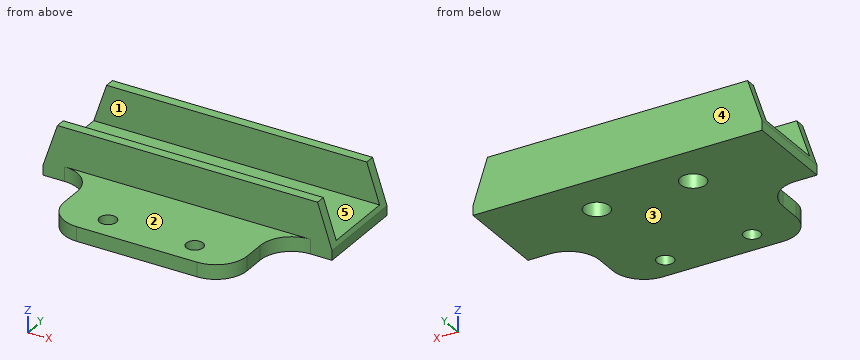
Autodesk Fusion 360 part; units mm, degrees
sketch "Esquisse1" plane through (0, 0, 0) normal (0, 0, 1) x (1, 0, 0)
  line L0 (0, 0) -> (60, 0)
  line L1 (60, 0) -> (60, 36.5)
  line L2 (60, 36.5) -> (0, 36.5)
  line L3 (0, 36.5) -> (0, 0)
  line L4 (0, 5) -> (60, 5) construction
  line L5 (0, 33.5) -> (60, 33.5) construction
  circle A0 centre (21, 5) radius 1.75
  circle A1 centre (39, 5) radius 1.75
  dimension "d1" = 28.5
  dimension "d2" = 60
  dimension "d3" = 18
  dimension "d4" = 21
  dimension "d5" = 3.5
  dimension "d6" = 5
  dimension "d7" = 3
extrude "Extrusion1" add sketch "Esquisse1" along normal blind 3
sketch "Esquisse2" plane through (0, 0, 3) normal (0, 0, 1) x (1, 0, 0)
  circle A0 centre (39, 5) radius 1.75
  circle A1 centre (21, 5) radius 1.75
  line L0 (0, 36.5) -> (0, 0)
  line L1 (0, 0) -> (60, 0)
  line L2 (60, 0) -> (60, 36.5)
  line L3 (60, 36.5) -> (0, 36.5)
  line L4 (0, 36.5) -> (60, 36.5)
  line L5 (60, 36.5) -> (60, 34.5)
  line L6 (60, 34.5) -> (0, 34.5)
  line L7 (0, 34.5) -> (0, 36.5)
  line L8 (0, 17.5) -> (60, 17.5)
  line L9 (60, 17.5) -> (60, 19.5)
  line L10 (60, 19.5) -> (0, 19.5)
  line L11 (0, 19.5) -> (0, 17.5)
  line L12 (60, 36.5) -> (0, 36.5)
  dimension "d10" = 15
  dimension "d11" = 2
  dimension "d12" = 2
extrude "Extrusion2" add sketch "Esquisse2" along normal blind 8 contours L0 L2 L3 L4 L5 L6 L7 L12 | L0 L2 L8 L9 L10 L11
sketch "Esquisse3" plane through (0, 0, 3) normal (0, 0, 1) x (1, 0, 0)
  line L0 (0, 19.5) -> (60, 19.5)
  line L1 (60, 19.5) -> (60, 34.5)
  line L2 (60, 34.5) -> (0, 34.5)
  line L3 (0, 34.5) -> (0, 19.5)
  line L4 (0, 27) -> (60, 27) construction
  circle A0 centre (20, 27) radius 2.625
  circle A1 centre (40, 27) radius 2.625
  line L5 (0, 36.5) -> (0, 0)
  dimension "d17" = 15
  dimension "d18" = 60
  dimension "d19" = 20
  dimension "d20" = 20
  dimension "d21" = 5.25
chamfer "Chanfrein2" distance 3 distance2 9 4 edges at (0, 18.5, 11) (0, 35.5, 11) (60, 35.5, 11) (60, 18.5, 11) measured on face at (20, 18.8333, 11) measured on face at (20, 35.1667, 11) measured on face at (20, 35.1667, 11) measured on face at (20, 18.8333, 11)
extrude "Extrusion3" cut sketch "Esquisse3" against normal blind 8 contours A0 | A1
sketch "Esquisse5" plane through (0, 0, 3) normal (0, 0, 1) x (1, 0, 0)
  line L0 (59.6667, 0) -> (59.6667, 17.5)
  line L1 (59.6667, 17.5) -> (0.3333, 17.5)
  line L2 (0.3333, 17.5) -> (0.3333, 0)
  line L3 (0.3333, 0) -> (59.6667, 0)
  circle A0 centre (39, 5) radius 1.75
  circle A1 centre (21, 5) radius 1.75
  line L4 (11, 0) -> (-11.5098, 0)
  line L5 (-11.5098, 0) -> (-11.5098, 17.5)
  line L6 (-11.5098, 17.5) -> (11, 17.5)
  line L7 (11, 17.5) -> (11, 0)
  line L8 (49, 0) -> (81.8509, 0)
  line L9 (81.8509, 0) -> (81.8509, 17.5)
  line L10 (81.8509, 17.5) -> (49, 17.5)
  line L11 (49, 17.5) -> (49, 0)
  point P0 (21, 5)
  point P1 (39, 5)
  dimension "d31" = 10
  dimension "d32" = 10
extrude "Extrusion5" cut sketch "Esquisse5" against normal blind 20 contours L0 L1 L3 L8 L10 L11 | L0 L8 L9 L10 | L1 L2 L3 L4 L6 L7 | L2 L4 L5 L6
fillet "Congé2" radius 6.5 4 edges at (11, 17.5, 1.5) (11, 0, 1.5) (49, 17.5, 1.5) (49, 0, 1.5)
equation "d4 = ( d2 - d3 ) / 2"
equation "d19 = d18 / 3"
equation "d20 = d19"
Geometry check sheet. Reference: the model listing, model coordinates, mm. Face numbers are marked on the shaded views. A direction names the side the tool comes from. Coordinates: 2 decimals unless noted, no trailing zeros. Loops run counter-clockwise (first coordinate to the right, second up) from the corner with the lowest first, then second, coordinate; pieces in that order, holes last.
Item 1: Sectioned sample at B-B, the plane x = 21. Record the boundary of the cut face in (y, z), then the cut area to 3 significant figures.
Item 2: Thickness scan on line 1 (Y direction, x = 21, z = 1.85); line 2 (Y direction, x = 40, z = 1.4) (3 decimals); line 3 (Y direction, x = 47.5, z = 10.5). Record the ranges inside material, lowest first.
Item 3: Release check for a two-part mould opening along Y. For the marked faces 3, 4 and 5 record: released by +Y, released by -Y, zero draft, split by the parting line, or undercut.
Item 4: Sectioned sample at D-D, the plane y = 25. Record the boundary of the cut face in (x, z), then the cut area to 3 significant figures.
Item 5: Go/stop test with flat-tipped pins: pin 1 Ø1.5 at (y, z) = (9.5, 1) entering from +X; pin 2 Ø4 at (y, z) = (13.5, 4.5) entering from -X; pin 3 Ø12 at (x, y) = (16, 23.5) entering from +Z; pin 4 Ø5.5 at (x, y) = (39, 5) entering from +Z. Record where each tip stops, or that it passes through.
Item 6: Sectioned sample at A-A, the plane z = 5. Record the boundary of the cut face in (x, y).
Item 7: Access from +Z, -Z, +X, -X, +Y, -Y to the whole of each face (thin tool, end or side, straight path). Record for the marked faces 1 and 2.
Item 8: Sectioned sample at C-C, the plane z = 1. Record the boundary of the cut face in (x, y) (3 decimals), then the cut area to 3 significant figures.
Check result:
1. outline: (0, 0) - (3.25, 0) - (3.25, 3) - (0, 3) - close; (6.75, 0) - (24.57, 0) - (24.57, 3) - (19.5, 3) - (19.5, 11) - (17.5, 11) - (17.5, 3) - (6.75, 3) - close; (29.43, 0) - (36.5, 0) - (36.5, 11) - (34.5, 11) - (34.5, 3) - (29.43, 3) - close
1. area: 116 mm2
2. line 1: y = 0 to 3.25, 6.75 to 24.57, 29.43 to 36.5
2. line 2: y = 0 to 3.564, 6.436 to 24.375, 29.625 to 36.5
2. line 3: y = 17.5 to 19.5, 34.5 to 36.5
3. face 3: zero draft
3. face 4: released by +Y
3. face 5: undercut
4. outline: (0, 0) - (18.3, 0) - (18.3, 3) - (0.33, 3) - (0, 2) - close; (21.7, 0) - (38.3, 0) - (38.3, 3) - (21.7, 3) - close; (41.7, 0) - (60, 0) - (60, 2) - (59.67, 3) - (41.7, 3) - close
4. area: 159 mm2
5. pin 1: stops at x = 49
5. pin 2: stops at x = 9.76
5. pin 3: stops at z = 11
5. pin 4: stops at z = 3
6. outline: (1, 17.5) - (59, 17.5) - (59, 19.5) - (1, 19.5) - close; (1, 34.5) - (59, 34.5) - (59, 36.5) - (1, 36.5) - close
7. face 1: +Z, +X, -X
7. face 2: +Z, +X, -X, -Y
8. outline: (0, 17.5) - (4.5, 17.5) arc R6.5 cw to (11, 11) - (11, 6.5) arc R6.5 ccw to (17.5, 0) - (42.5, 0) arc R6.5 ccw to (49, 6.5) - (49, 11) arc R6.5 cw to (55.5, 17.5) - (60, 17.5) - (60, 36.5) - (0, 36.5) - close; hole circle Ø5.25 at (20, 27); hole circle Ø3.5 at (21, 5); hole circle Ø3.5 at (39, 5); hole circle Ø5.25 at (40, 27)
8. area: 1,740 mm2
